Design review of the part built by this model. Coordinates are the model's own, in mm. Face numbers are marked on the shaded views. Give positions to 0.01 mm unless a question says otherwise; leave off trailing zeros. Order: outer loops, then holes, each group sorted by start corner. A loop starts at its lowest first (then second) coordinate and runs counter-clockwise, first axis right, second up. Notation, with made-up numbers: (78, -39) -> (123, -39) arc R9 ccw to (123, -31) -> close; hole circle Ø10 at (74, 74). An arc over 180 degrees is marked (long way). Use a Markdown table: item, result. Add a question column.
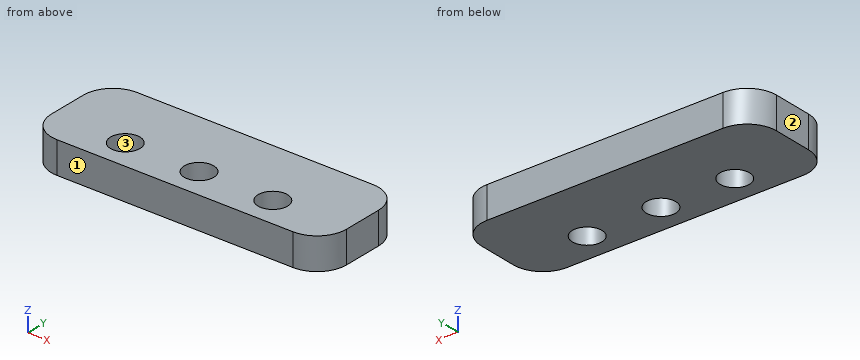
```python
from build123d import *

# Parameters (mm, degrees)
SKETCH1_W           = 30
SKETCH1_H           = 10
SKETCH1_R           = 1.5
BOSS_EXTRUDE1_DEPTH = 1.61
FILLET1_R           = 3


with BuildPart() as part:
    # Sketch1 → Boss-Extrude1 (new body, symmetric)
    with BuildSketch(Plane.XY):
        with Locations((0, 2)):
            Rectangle(SKETCH1_W, SKETCH1_H)
        with Locations((-7.5, 0)):
            Circle(SKETCH1_R, mode=Mode.SUBTRACT)
        Circle(SKETCH1_R, mode=Mode.SUBTRACT)
        with Locations((7.5, 0)):
            Circle(SKETCH1_R, mode=Mode.SUBTRACT)
    extrude(amount=BOSS_EXTRUDE1_DEPTH, both=True)

    # Fillet1
    fillet1_edges = [part.edges().sort_by_distance(p)[0] for p in [
        (15, -3, 0),
        (-15, -3, 0),
        (-15, 7, 0),
        (15, 7, 0),
    ]]
    fillet(fillet1_edges, radius=FILLET1_R)


solid = part.part
```
1) Add section B-B (z = -0.2). Give the boundary of the cut face in (x, y).
2) Add section A-A (x = 0). Give the boundary of the cut face in (y, z).
3) The part is to be moulded in two halves that separate along X. For the marked faces 1, 2 and 3, say which applies: +X half, -X half, draft (parallel to the pull), parting line (faces both ways), or undercut.
4) Add section C-C (x = -13). Give the boundary of the cut face in (y, z).
5) For L1, parallel to Y at x = 0, z = -0.2; L2, parallel to X at y = 0.25, z = -0.55; L3, parallel to Y at x = 8, z = -0.75, list the stretches that pass through material, from the lowest coordinate up. Write a range as [from, to].
Worked answers:
| question | item | result |
|---|---|---|
| 1 | outline | (-15, 0) arc R3 ccw to (-12, -3) -> (12, -3) arc R3 ccw to (15, 0) -> (15, 4) arc R3 ccw to (12, 7) -> (-12, 7) arc R3 ccw to (-15, 4) -> close; hole circle Ø3 at (-7.5, 0); hole circle Ø3 at (0, 0); hole circle Ø3 at (7.5, 0) |
| 2 | outline | (-3, -1.61) -> (-1.5, -1.61) -> (-1.5, 1.61) -> (-3, 1.61) -> close; (1.5, -1.61) -> (7, -1.61) -> (7, 1.61) -> (1.5, 1.61) -> close |
| 3 | face 1 | draft |
| 3 | face 2 | -X half |
| 3 | face 3 | undercut |
| 4 | outline | (-2.83, -1.61) -> (6.83, -1.61) -> (6.83, 1.61) -> (-2.83, 1.61) -> close |
| 5 | L1 | [-3, -1.5], [1.5, 7] |
| 5 | L2 | [-15, -8.98], [-6.02, -1.48], [1.48, 6.02], [8.98, 15] |
| 5 | L3 | [-3, -1.41], [1.41, 7] |
